Model file for the job. Use its own axes, mm. Give positions to 0.01 mm unless a question says otherwise; leave off trailing zeros. Loops run counter-clockwise (first coordinate to the right, second up) from the corner with the lowest first, then second, coordinate; pieces in that order, holes last. Notation, with made-up numbers: (52.25, -32) - (79.25, -32) arc R24 cw to (79.25, -20) - close; hole circle Ø10 at (64, 22.25). An arc over 180 degrees is marked (long way). Answer as CSV lines item,"result". Start each with the question number.
Item 1: Saw through at A-A on y = 3.75. Give the cut face in (x, z), plus the area to 3 significant figures.
Item 2: Saw through at B-B on z = -0.5. Give the cut face in (x, y).
Item 3: Saw through at C-C on x = 1.65. Give the cut face in (y, z).
Item 4: Saw through at D-D on y = 5.75. Give the cut face in (x, z).
Item 5: Drill centre lines: L1, parallel to Y at x = 0.9, z = 0; L2, parallel to Y at x = 1.3, z = 1.75. Where is each one in solid material? Low to high. Write a range as from..to.
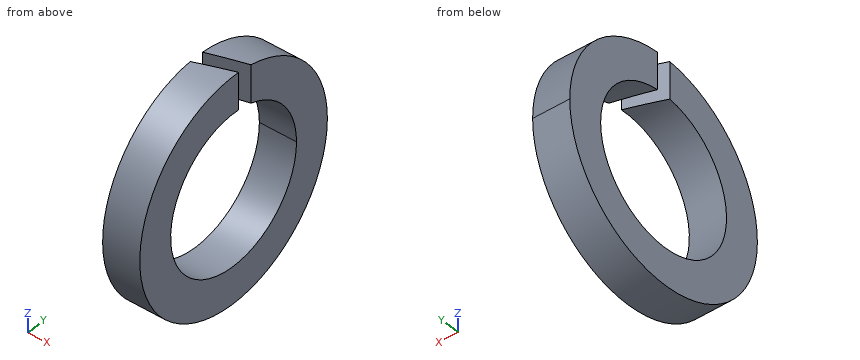
Autodesk Inventor part; units mm, degrees
ref_plane "Work Plane1" through (0, 0, 0) normal (0, -1, 0) x (1, 0, 0)
ref_plane "YZ Plane" through (0, 0, 0) normal (1, 0, 0) x (0, 1, 0)
ref_plane "XZ Plane" through (0, 0, 0) normal (0, 1, 0) x (-1, 0, 0)
sketch "Эскиз1" plane through (0, 0, 0) normal (1, 0, 0) x (0, 1, 0)
  circle A0 centre (0, 0) radius 7.6
  circle A1 centre (0, 0) radius 5.1
  dimension "d0" = 10.2
  dimension "d1" = 15.2
extrude "Базовый элемент" add sketch "Эскиз1" along normal blind 2.5
sketch "Эскиз2" plane through (0, 0, 0) normal (0, 0, 1) x (1, 0, 0)
  line L0 (0, -5.1) -> (0, 5.1)
  line L1 (2.5, 7.6) -> (2.5, -7.6)
  line L2 (-1.2, 0) -> (7.2, 0)
  line L3 (0, -0.5) -> (2.5, 0.4099)
  line L4 (0, 0.5) -> (2.5, 1.4099)
  dimension "d4" = 0.5
  dimension "d5" = 0.5
  dimension "d6" = 70
extrude "Вырез" cut sketch "Эскиз2" along normal up to next contours L0 L2 L3 | L0 L4 L1 L3 L2
ref_plane "Work Plane1" through (0, 0, 0) normal (0, -1, 0) x (1, 0, 0)
equation "\"d0\" = SD1"
equation "\"d1\" = SD2"
equation "\"d2\" = SD"
equation "\"d4\" = 0.2 * SD"
equation "\"d5\" = 0.2 * SD"
equation "\"d6\" = FAWI"
equation "\"d7\" = SD"
equation "\"SD1\" = 10.2"
equation "\"SD2\" = 15.2"
equation "\"SD\" = 2.5"
equation "\"FAWI\" = 70deg"
properties part number "Шайба  10 N ГОСТ 6402-70" material "Сталь, мягкая"
Responses:
1,outline,"(0, -6.61) - (2.5, -6.61) - (2.5, -3.46) - (0, -3.46) - close; (0, 3.46) - (2.5, 3.46) - (2.5, 6.61) - (0, 6.61) - close"
1,area,"15.8 mm2"
2,outline,"(0, -7.58) - (2.5, -7.58) - (2.5, -5.08) - (0, -5.08) - close; (0, 5.08) - (2.5, 5.08) - (2.5, 7.58) - (0, 7.58) - close"
3,outline,"(0.1, 5.1) - (0.1, 7.6) arc R7.6 ccw (long way) to (1.1, 7.52) - (1.1, 4.98) arc R5.1 cw (long way) to start"
4,outline,"(0, -4.97) - (2.5, -4.97) - (2.5, 4.97) - (0, 4.97) - close"
5,L1,"-7.6..-5.1, 5.1..7.6"
5,L2,"-7.4..-4.79, 4.79..7.4"
